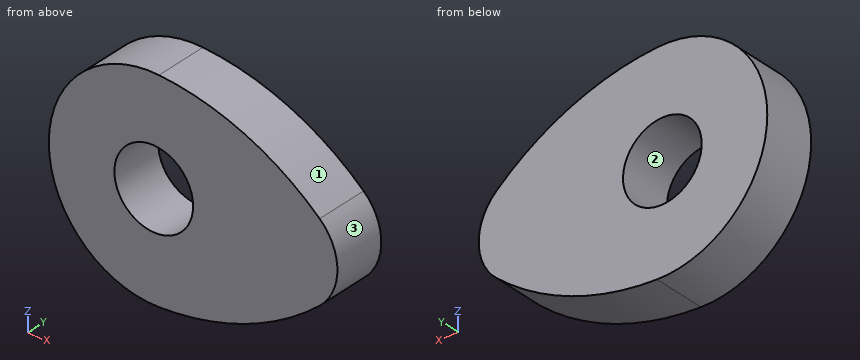
```python
from build123d import *

# Parameters (mm, degrees)
SKETCH1_R           = 7.5
BOSS_EXTRUDE1_DEPTH = 5


with BuildPart() as part:
    # Sketch1 → Boss-Extrude1 (new, symmetric)
    with BuildSketch(Plane(origin=(0, 0, 0), x_dir=(1, 0, 0), z_dir=(0, 1, 0))):
        with BuildLine():
            ThreePointArc((1, 19.974984355), (-20, 0), (1, -19.974984355))
            ThreePointArc((1, -19.974984355), (17.374586088, -16.33817141), (31.625, -7.490619133))
            ThreePointArc((31.625, -7.490619133), (35, 0), (31.625, 7.490619133))
            ThreePointArc((31.625, 7.490619133), (17.374586088, 16.33817141), (1, 19.974984355))
        make_face()
        with Locations(Location((0, 0, 0), (0, 0, 270))):
            Circle(SKETCH1_R, mode=Mode.SUBTRACT)
    extrude(amount=BOSS_EXTRUDE1_DEPTH, both=True)


solid = part.part
```
Here's how the part is built. I have some questions about the finished solid (model axes, mm). Face numbers are marked on the shaded views. Coordinates: 2 decimals unless noted, no trailing zeros. Loops run counter-clockwise (first coordinate to the right, second up) from the corner with the lowest first, then second, coordinate; pieces in that order, holes last. Notation, with made-up numbers: (76, -16) - (117, -16) arc R23 ccw to (117, 1) - close; hole circle Ø4 at (40.5, 83). An arc over 180 degrees is marked (long way). Answer as CSV lines item,"result".
Q1. If we section it at A-A, the plane x = 0: Write out the boundary of the cut face in (y, z).
Response:
outline,"(-5, -20) - (5, -20) - (5, -7.5) - (-5, -7.5) - close; (-5, 7.5) - (5, 7.5) - (5, 20) - (-5, 20) - close"
Q2. If we section it at D-D, the plane x = -16: Write out the boundary of the cut face in (y, z), and give its area (3 significant figures).
Response:
outline,"(-5, -12) - (5, -12) - (5, 12) - (-5, 12) - close"
area,"240 mm2"
Q3. For pin 1 (1.5 mm diameter, centred on x = -11, y = -1.5, fed in from +Z); pin 2 (19.5 mm diameter, centred on x = 0, z = 0, fed in from +Y); pin 3 (3 mm diameter, centred on y = 3.5, z = 12.5, fed in from +X), each with a flat end and sliding along its axis, tell me the tip position at first contact or that it passes through.
Response:
pin 1,"z = 17.17"
pin 2,"y = 5"
pin 3,"x = 27.17"
Q4. If we section it at B-B, the plane z = 0: Write out the boundary of the cut face in (x, y), and give its area (3 significant figures).
Response:
outline,"(-20, -5) - (-7.5, -5) - (-7.5, 5) - (-20, 5) - close; (7.5, -5) - (35, -5) - (35, 5) - (7.5, 5) - close"
area,"400 mm2"
Q5. We'd pull the mould along Z, two halves only. Please class the marked faces 1, 2 and 3: pulls with the +Z half, pulls with the -Z half, needs draft (parallel to the pull), parting line crosses it, or undercut.
Response:
face 1,"pulls with the +Z half"
face 2,"undercut"
face 3,"parting line crosses it"
Q6. If I drill on L1, parallel to X at y = -1.5, z = 0; L2, parallel to X at y = 3.5, z = -2; L3, parallel to Z at x = -5.5, y = 1.5, over which ranges is the centre line in solid material (lowest first)? Write a range as [from, to].
Response:
L1,"[-20, -7.5], [7.5, 35]"
L2,"[-19.9, -7.23], [7.23, 34.8]"
L3,"[-19.23, -5.1], [5.1, 19.23]"
Q7. If we section it at C-C, the plane y = -3.25: Write out the boundary of the cut face in (x, z) (3 decimals), and give its area (3 significant figures).
Response:
outline,"(1, -19.975) arc R50 ccw to (31.625, -7.491) arc R10 ccw to (31.625, 7.491) arc R50 ccw to (1, 19.975) arc R20 ccw (long way) to start; hole circle Ø15 at (0, 0)"
area,"1,490 mm2"
